Can you work these out from the model? Positions are in its coordinate system, mm. A direction names the side the tool comes from. Coordinates: 2 decimals unless noted, no trailing zeros. Loops run counter-clockwise (first coordinate to the right, second up) from the corner with the lowest first, then second, coordinate; pieces in that order, holes last. Notation, with made-up numbers: M -24.75,78 L 9.25,78 A35 cw 9.25,116 Z; hole C 37.5,82 d6. An arc over 180 degrees is marked long. Answer as a JSON object with one key per item and string values. Group by question number.
Item 1: If I drill on line 1 (X direction, y = 2.75, z = -11); line 2 (Z direction, x = -11, y = 1); line 3 (Z direction, x = -9.25, y = 0.5), over which ranges is the centre line in solid material (lowest first)?
Item 2: Suppose I cut it at C-C (x = 0). Write out the boundary of the cut face in (y, z), then the cut area to 4 significant figures.
Item 3: Suppose I cut it at B-B (y = 3.5). Write out the boundary of the cut face in (x, z).
Item 4: Suppose I cut it at A-A (z = -4). Write out the boundary of the cut face in (x, y).
Item 5: We'd pull the mould along Z, two halves only. Please class faces 5 (the cylindrical face through (0.33, 1.972, -47.496)), 6 (the flat face through (0, 2, 0)), 7 (the flat face through (1.5, 7, -4)), 8 (the cylindrical face through (-0.26, 2.77, -9.83)): +Z half, -Z half, draft (parallel to the pull), parting line (faces both ways), or undercut.
Item 6: Which directions (+Z, -Z, +X, -X, +Y, -Y) give clear straight access to the entire face, cutting with the end or side of a thin tool? Please do faces 1 (the flat face through (0, 7, -2.5)), 2 (the flat face through (0, 7, -5.5)), 3 (the flat face through (-1.5, 7, -4)), 4 (the cylindrical face through (0.55, 2.028, -44.988)).
Item 7: I'm going to push flat-ended pins straight in: pin 1 Ø3.5 at (x, y) = (0.5, 6) entering from +Z; pin 2 Ø1.5 at (y, z) = (6.5, -4) entering from -X; pin 3 Ø6 at (x, y) = (-0.5, 4) entering from -Z; pin 4 Ø4 at (x, z) = (10, -4) entering from +Y. Where does each tip first touch, or does it pass through?
Item 8: Suppose I cut it at D-D (z = -11). Write out the boundary of the cut face in (x, y).
```python
from build123d import *

# Parameters (mm, degrees)
BOSS_EXTRUDE1_DEPTH                                 = 4
CUT_EXTRUDE1_REACH                                  = 51.972
SKETCH2_R                                           = 12.5
SKETCH3_W                                           = 3
SKETCH3_H                                           = 3
BOSS_EXTRUDE2_DEPTH                                 = 6
CSK_FOR_M2_COUNTERSUNK_FLAT_HEAD_SCREW1_D           = 2.4
CSK_FOR_M2_COUNTERSUNK_FLAT_HEAD_SCREW1_DEPTH       = 5.2
CSK_FOR_M2_COUNTERSUNK_FLAT_HEAD_SCREW1_CSINK_D     = 5.4
CSK_FOR_M2_COUNTERSUNK_FLAT_HEAD_SCREW1_CSINK_ANGLE = 90
CSK_FOR_M2_COUNTERSUNK_FLAT_HEAD_SCREW1_TIP         = 0.721032743


with BuildPart() as part:
    # Sketch1 → Boss-Extrude1 (new body)
    with BuildSketch(Plane(origin=(0, 0, 0), x_dir=(1, 0, 0), z_dir=(0, 1, 0))):
        with BuildLine():
            Line((-15, 0), (15, 0))
            Line((15, 0), (15, 32.5))
            ThreePointArc((15, 32.5), (0, 47.5), (-15, 32.5))
            Line((-15, 32.5), (-15, 0))
        make_face()
    extrude(amount=BOSS_EXTRUDE1_DEPTH)

    # Sketch2 → Cut-Extrude1 (cut, up to next)
    with BuildSketch(Plane(origin=(0, 4, 0), x_dir=(1, 0, 0), z_dir=(0, 1, 0)), mode=Mode.PRIVATE) as cut_extrude1_sk1:
        with Locations(Location((0, 32.5, 0), (0, 0, 270))):
            Circle(SKETCH2_R)
    cut_extrude1_tool1 = extrude(cut_extrude1_sk1.sketch, amount=-CUT_EXTRUDE1_REACH, mode=Mode.PRIVATE) & part.part
    add(cut_extrude1_tool1.solids().sort_by_distance((0, 4, -32.5))[0], mode=Mode.SUBTRACT)

    # Sketch3 → Boss-Extrude2 (add)
    with BuildSketch(Plane(origin=(0, 4, 0), x_dir=(1, 0, 0), z_dir=(0, 1, 0))):
        with Locations((0, 4)):
            Rectangle(SKETCH3_W, SKETCH3_H)
    extrude(amount=BOSS_EXTRUDE2_DEPTH)

    # CSK for M2 Countersunk Flat Head Screw1
    with Locations(Plane(origin=(0, 0, 0), x_dir=(-1, 0, 0), z_dir=(0, -1, 0))):
        with Locations((-10, 4), (10, 4), (0, 11)):
            CounterSinkHole(CSK_FOR_M2_COUNTERSUNK_FLAT_HEAD_SCREW1_D / 2, CSK_FOR_M2_COUNTERSUNK_FLAT_HEAD_SCREW1_CSINK_D / 2, depth=CSK_FOR_M2_COUNTERSUNK_FLAT_HEAD_SCREW1_DEPTH, counter_sink_angle=CSK_FOR_M2_COUNTERSUNK_FLAT_HEAD_SCREW1_CSINK_ANGLE)
            with Locations((0, 0, -(CSK_FOR_M2_COUNTERSUNK_FLAT_HEAD_SCREW1_DEPTH + CSK_FOR_M2_COUNTERSUNK_FLAT_HEAD_SCREW1_TIP / 2))):  # 118° drill point
                Cone(0, CSK_FOR_M2_COUNTERSUNK_FLAT_HEAD_SCREW1_D / 2, CSK_FOR_M2_COUNTERSUNK_FLAT_HEAD_SCREW1_TIP, mode=Mode.SUBTRACT)


solid = part.part
```
From the geometry:
{
 "1": {"line 1": "-15 to -1.2, 1.2 to 15", "line 2": "-42.7 to -38.44, -26.56 to -5.37, -2.63 to 0", "line 3": "-44.31 to -40.91, -24.09 to -6.07, -1.93 to 0"},
 "2": {"outline": "M 0,-47.5 L 4,-47.5 L 4,-45 L 0,-45 Z; M 0,-20 L 4,-20 L 4,-12.2 L 1.5,-12.2 L 0,-13.7 Z; M 0,-8.3 L 1.5,-9.8 L 4,-9.8 L 4,-5.5 L 10,-5.5 L 10,-2.5 L 4,-2.5 L 4,0 L 0,0 Z", "area": "96.15 mm2"},
 "3": {"outline": "M -15,-32.5 A15 ccw 15,-32.5 L 15,0 L -15,0 Z; hole C 0,-32.5 d25; hole C -10,-4 d2.4; hole C 0,-11 d2.4; hole C 10,-4 d2.4"},
 "4": {"outline": "M -15,0 L -12.7,0 L -11.2,1.5 L -11.2,4 L -15,4 Z; M -8.8,1.5 L -7.3,0 L 7.3,0 L 8.8,1.5 L 8.8,4 L 1.5,4 L 1.5,10 L -1.5,10 L -1.5,4 L -8.8,4 Z; M 11.2,1.5 L 12.7,0 L 15,0 L 15,4 L 11.2,4 Z"},
 "5": {"face 5": "-Z half", "face 6": "+Z half", "face 7": "draft", "face 8": "undercut"},
 "6": {"face 1": "+Z, +X, -X, +Y", "face 2": "-Z, +X, -X, +Y", "face 3": "+Z, -Z, -X, +Y", "face 4": "+Y, -Y"},
 "7": {"pin 1": "z = -2.5", "pin 2": "x = -1.5", "pin 3": "z = -47.5", "pin 4": "y = 4"},
 "8": {"outline": "M -15,0 L -2.7,0 L -1.2,1.5 L -1.2,4 L -15,4 Z; M 1.2,1.5 L 2.7,0 L 15,0 L 15,4 L 1.2,4 Z"}
}
